Autodesk Inventor part; units mm, degrees
ref_plane "YZ Plane" through (0, 0, 0) normal (1, 0, 0) x (0, 1, 0)
ref_plane "XZ Plane" through (0, 0, 0) normal (0, 1, 0) x (-1, 0, 0)
ref_plane "XY Plane" through (0, 0, 0) normal (0, 0, 1) x (1, 0, 0)
sketch "Sketch1" plane through (0, 0, 0) normal (0, 0, 1) x (1, 0, 0)
  line L0 (0, 0) -> (37.5, 0) construction
  line L1 (0, -10) -> (37.5, -10)
  line L2 (37.5, 10) -> (0, 10)
  arc A0 (0, 10) -> (0, -10) centre (0, 0) ccw
  arc A1 (37.5, -10) -> (37.5, 10) centre (37.5, 0) ccw
  line L3 (0, 0) -> (37.5, 0) construction
  circle A2 centre (0, 0) radius 1.5
  circle A3 centre (37.5, -5) radius 1.5
  circle A4 centre (37.5, 5) radius 1.5
  point P0 (18.75, 0)
  dimension "d0" = 37.5
  dimension "d1" = 0
  dimension "d2" = 20
  dimension "d3" = 3
  dimension "d4" = 3
  dimension "d5" = 3
  dimension "d6" = 10
  dimension "d7" = 5
  dimension "d8" = 0
  dimension "d9" = 0
extrude "Extrusion1" add sketch "Sketch1" along normal blind 3
sketch "Sketch2" plane through (0, 0, 0) normal (0, 0, -1) x (-1, 0, 0)
  line L0 (6, 5) -> (-25, 5)
  line L1 (-25, 10) -> (-25, -10)
  line L2 (-25, -5) -> (6, -5)
  line L3 (6, -5) -> (6, 5)
  arc A0 (-37.5, 10) -> (-37.5, -10) centre (-37.5, 0) ccw
  line L4 (0, -10) -> (-37.5, -10)
  arc A1 (0, -10) -> (0, 10) centre (0, 0) ccw
  line L5 (-37.5, 10) -> (0, 10)
  circle A2 centre (-37.5, 5) radius 1.5
  circle A3 centre (-37.5, -5) radius 1.5
  circle A4 centre (0, 0) radius 1.5
  dimension "d12" = 6
  dimension "d13" = 5
  dimension "d14" = 5
  dimension "d15" = 25
extrude "Extrusion2" cut sketch "Sketch2" against normal up to surface (3 mm away) contours L0 L1 L5 A1 L4 L2 L3
fillet "Fillet1" radius 2.5 4 edges at (25, 5, 1.5) (25, 10, 1.5) (25, -5, 1.5) (25, -10, 1.5)
fillet "Fillet2" radius 5 2 edges at (-6, 5, 1.5) (-6, -5, 1.5)
sketch "Sketch3" plane through (0, 0, 3) normal (0, 0, 1) x (1, 0, 0)
  arc A0 (-1, 5) -> (-1, -5) centre (-1, 0) ccw
  line L0 (-1, -5) -> (22.5, -5)
  arc A1 (25, -7.5) -> (22.5, -5) centre (22.5, -7.5) ccw
  arc A2 (25, -7.5) -> (27.5, -10) centre (27.5, -7.5) ccw
  line L1 (27.5, -10) -> (37.5, -10)
  arc A3 (37.5, -10) -> (37.5, 10) centre (37.5, 0) ccw
  line L2 (37.5, 10) -> (27.5, 10)
  arc A4 (27.5, 10) -> (25, 7.5) centre (27.5, 7.5) ccw
  arc A5 (22.5, 5) -> (25, 7.5) centre (22.5, 7.5) ccw
  line L3 (22.5, 5) -> (-1, 5)
  circle A6 centre (37.5, 5) radius 1.5
  circle A7 centre (37.5, -5) radius 1.5
  circle A8 centre (0, 0) radius 1.5
properties part number "Arm5_3D" material "Aluminum 6061, Welded"
Part model, mm, in its own coordinate system. A direction names the side the tool comes from. Round coordinates to 2 decimals unless told otherwise and drop trailing zeros. Write each loop counter-clockwise with the first axis right and the second up, starting at its lowest first coordinate (ties: lowest second). Pieces come first, ordered by that corner, then holes. Notation, with made-up numbers: (26, 67) - (44, 67) arc R19 cw to (44, 82) - close; hole circle Ø5 at (25.25, 73.5). An arc over 180 degrees is marked (long way). Use CSV: the item, a comma, the result in double quotes.
Item 1: Slice it at C-C, the plane z = 1.1. Count the separate pieces of the cut face and the enclosed holes in it, then the cut area to 3 significant figures.
Results list:
separate pieces,"1"
enclosed holes,"3"
area,"685 mm²"
Item 2: Flat gauge pins, fed straight in: P1, Ø1.5, axis at x = 9.5, z = 2, coming from the +Y side; P2, Ø1.5, axis at x = 20.5, y = -7, coming from the -Z side. Where does each tip first touch, or does it go through?
Results list:
P1,"stops at y = 5"
P2,"passes through"
Item 3: Slice it at D-D, the plane x = 15. Write the cut outline in (y, z), then the cut area to 3 significant figures.
Results list:
outline,"(-5, 0) - (5, 0) - (5, 3) - (-5, 3) - close"
area,"30.0 mm²"
Item 4: Slice it at B-B, the plane y = -6. Write the cut outline in (x, z), then the cut area to 3 significant figures.
Results list:
outline,"(24.5, 0) - (36.38, 0) - (36.38, 3) - (24.5, 3) - close; (38.62, 0) - (45.5, 0) - (45.5, 3) - (38.62, 3) - close"
area,"56.3 mm²"
Item 5: Slice it at A-A, the plane x = 0. Write the cut outline in (y, z), then the cut area to 3 significant figures.
Results list:
outline,"(-5, 0) - (-1.5, 0) - (-1.5, 3) - (-5, 3) - close; (1.5, 0) - (5, 0) - (5, 3) - (1.5, 3) - close"
area,"21.0 mm²"
Item 6: Wall check: L1, parallel to Y at x = 37.5, z = 2.3; L2, parallel to Y at x = 0, z = 2.3; L3, parallel to Y at x = 6.5, z = 1.5. Give the ranges that are in metal, low to high.
Results list:
L1,"y = -10 to -6.5, -3.5 to 3.5, 6.5 to 10"
L2,"y = -5 to -1.5, 1.5 to 5"
L3,"y = -5 to 5"
Item 7: Tool access for faces 1 (the flat face through (11, 5, 1)), 2 (the flat face through (26, 0, 3)), 3 (the flat face through (11, -5, 1)): list every direction of +Z, -Z, +X, -X, +Y, -Y with a clear straight run to the whole face (end or side of a thin tool).
Results list:
face 1,"+Z, -Z, -X, +Y"
face 2,"+Z, +X, -X, +Y, -Y"
face 3,"+Z, -Z, -X, -Y"
